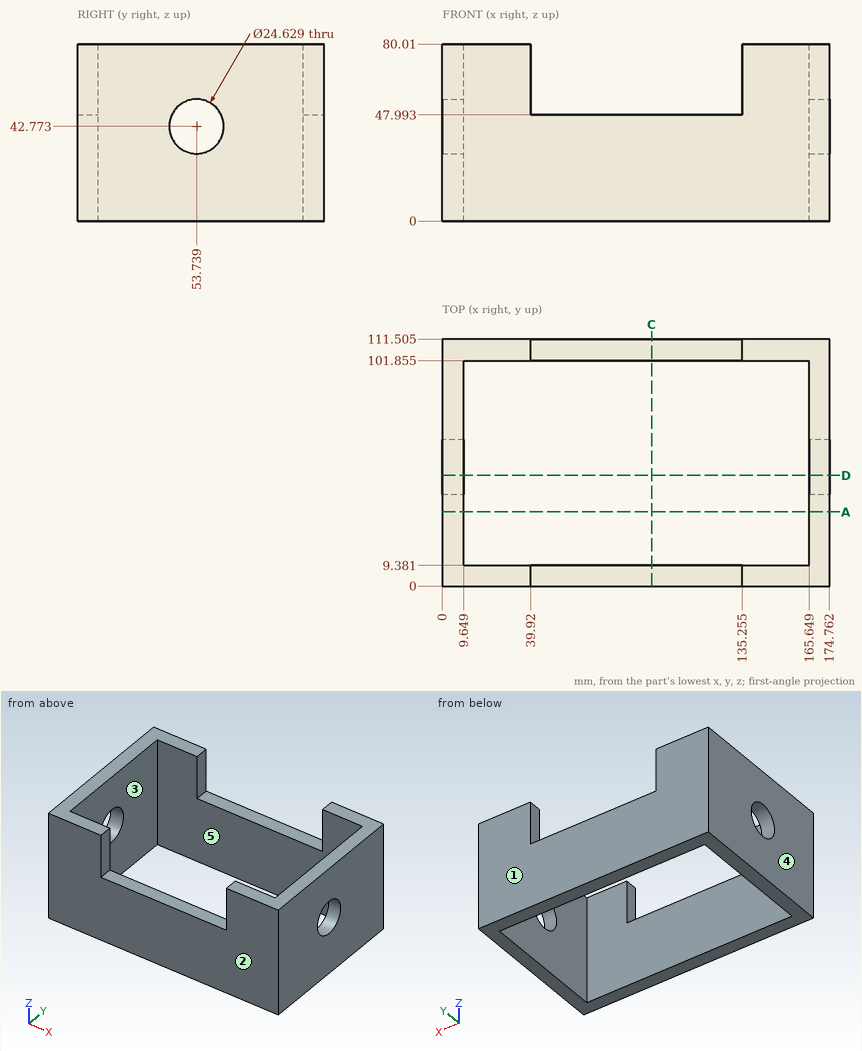
The drawing under review shows one solid part. Ordinate dimensions are in mm from its lowest x, y, z. A direction names the side the tool comes from. Give positions to 0.01 mm unless a question says otherwise; leave off trailing zeros. Write each loop counter-clockwise with the first axis right and the second up, starting at its lowest first coordinate (ties: lowest second). Pieces come first, ordered by that corner, then holes. Notation, with made-up numbers: (-23.75, 13.5) - (-2.75, 13.5) arc R29 ccw to (-2.75, 41.5) - close; hole circle Ø4 at (76, 56.25). An arc over 180 degrees is marked (long way). Answer in a Markdown table with one row per item. Add a question column.
1. We need section C-C on x = 94.5. Write out the cut boundary in (y, z) (1 decimal).
2. Tool access review of the marked faces 4 and 5: name each direction out of +Z, -Z, +X, -X, +Y, -Y from which nothing blocks a thin tool from reaching the whole face with its end or side.
3. We need section D-D on y = 50. State how many separate pieces and enclosed holes the cut face has, then the cut area to 3 significant figures.
4. Insertion check: P1, Ø4.5, axis at x = 90.5, y = 5.5, coming from the +Z side; P2, Ø19.5, axis at y = 53.74, z = 42.77, coming from the -X side. Each pin has a flat end and moves straight along its axis. Give the tip position at first contact, or say it passes through.
5. Wall thickness on line 1 along X through (y, z) = (87, 10); line 2 along Y through (x, z) = (124.5, 30) (1 decimal); line 3 along X through (y, z) = (102, 72) (1 decimal): over which ranges is each line inside the solid? List them lowest first. Write a range as [from, to].
6. We need section A-A on y = 33.5. Write out the cut boundary in (x, z).
7. Draft analysis for pull direction Y (two halves, no side actions). For the marked faces 1, 2 and 3, state which applies: +Y half, -Y half, draft (parallel to the pull), parting line (faces both ways), or undercut.
Ans:
| question | item | result |
|---|---|---|
| 1 | outline | (0, 0) - (9.4, 0) - (9.4, 48) - (0, 48) - close; (101.9, 0) - (111.5, 0) - (111.5, 48) - (101.9, 48) - close |
| 2 | face 4 | +Z, -Z, -X, +Y, -Y |
| 2 | face 5 | +Z, -Z |
| 3 | separate pieces | 4 |
| 3 | enclosed holes | 0 |
| 3 | area | 1,060 mm^2 |
| 4 | P1 | stops at z = 47.99 |
| 4 | P2 | passes through |
| 5 | line 1 | x = [0, 9.65], [165.65, 174.76] |
| 5 | line 2 | y = [0, 9.4], [101.9, 111.5] |
| 5 | line 3 | x = [0, 39.9], [135.3, 174.8] |
| 6 | outline | (0, 0) - (9.65, 0) - (9.65, 80.01) - (0, 80.01) - close; (165.65, 0) - (174.76, 0) - (174.76, 80.01) - (165.65, 80.01) - close |
| 7 | face 1 | +Y half |
| 7 | face 2 | -Y half |
| 7 | face 3 | undercut |
